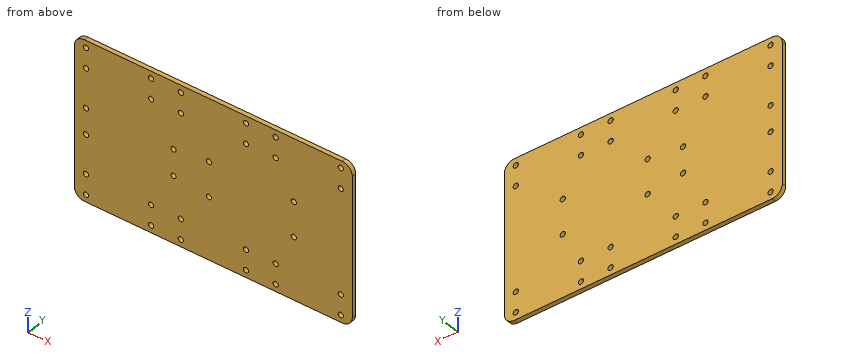
from build123d import *

# Parameters (mm, degrees)
SKETCH1_W            = 190
SKETCH1_H            = 110
BOSS_EXTRUDE1_DEPTH  = 3
M3_CLEARANCE_HOLE1_D = 3.6
FILLET1_R            = 7


with BuildPart() as part:
    # Sketch1 → Boss-Extrude1 (new body)
    with BuildSketch(Plane(origin=(0, 0, 0), x_dir=(1, 0, 0), z_dir=(0, 1, 0))):
        with Locations((95, 55)):
            Rectangle(SKETCH1_W, SKETCH1_H)
    extrude(amount=BOSS_EXTRUDE1_DEPTH)

    # M3 Clearance Hole1 (through all)
    with Locations(Plane(origin=(0, 3, 0), x_dir=(1, 0, 0), z_dir=(0, 1, 0))):
        with Locations((8, 105), (52.5, 105), (52.5, 91), (8, 91), (52.5, 19), (52.5, 5), (8, 19), (8, 5), (72.811, 105), (117.311, 105), (117.311, 91), (72.811, 91), (137.622, 105), (182.122, 105), (182.122, 91), (137.622, 91), (72.811, 19), (117.311, 19), (137.622, 19), (182.122, 19), (182.122, 5), (137.622, 5), (117.311, 5), (72.811, 5), (8, 64), (8, 46), (67.78, 64), (67.78, 46), (92, 67), (92, 43), (150, 43), (150, 67)):
            Hole(M3_CLEARANCE_HOLE1_D / 2)

    # Fillet1
    fillet1_edges = [part.edges().sort_by_distance(p)[0] for p in [
        (0, 1.5, -110),
        (190, 1.5, -110),
        (190, 1.5, 0),
        (0, 1.5, 0),
    ]]
    fillet(fillet1_edges, radius=FILLET1_R)


solid = part.part
For this review, take the finished solid that the model builds, in its own axes (mm). Round coordinates to 2 decimals unless told otherwise and drop trailing zeros. Order: outer loops, then holes, each group sorted by start corner. A loop starts at its lowest first (then second) coordinate and runs counter-clockwise, first axis right, second up. Notation, with made-up numbers: (-31, 36.5) -> (-15, 36.5) arc R21 cw to (-15, 66.5) -> close; hole circle Ø7 at (-4, 87). An arc over 180 degrees is marked (long way). Put each result on its own line as item: value.
Q1. For probe 1 along Z at (x, y) = (73, 0.8); probe 2 along X at (y, z) = (1.6, -67); probe 3 along X at (y, z) = (2.3, -64), list the stretches that pass through material, from the lowest coordinate up. Write a range as [from, to].
Check result:
probe 1: [-110, -106.79], [-103.21, -92.79], [-89.21, -20.79], [-17.21, -6.79], [-3.21, 0]
probe 2: [0, 90.2], [93.8, 148.2], [151.8, 190]
probe 3: [0, 6.2], [9.8, 65.98], [69.58, 190]
Q2. Add section D-D on z = -105. Write out the cut boundary in (x, y).
Check result:
outline: (0.29, 0) -> (6.2, 0) -> (6.2, 3) -> (0.29, 3) -> close; (9.8, 0) -> (50.7, 0) -> (50.7, 3) -> (9.8, 3) -> close; (54.3, 0) -> (71.01, 0) -> (71.01, 3) -> (54.3, 3) -> close; (74.61, 0) -> (115.51, 0) -> (115.51, 3) -> (74.61, 3) -> close; (119.11, 0) -> (135.82, 0) -> (135.82, 3) -> (119.11, 3) -> close; (139.42, 0) -> (180.32, 0) -> (180.32, 3) -> (139.42, 3) -> close; (183.92, 0) -> (189.71, 0) -> (189.71, 3) -> (183.92, 3) -> close
Q3. Add section A-A on z = -19. Write out the cut boundary in (x, y).
Check result:
outline: (0, 0) -> (6.2, 0) -> (6.2, 3) -> (0, 3) -> close; (9.8, 0) -> (50.7, 0) -> (50.7, 3) -> (9.8, 3) -> close; (54.3, 0) -> (71.01, 0) -> (71.01, 3) -> (54.3, 3) -> close; (74.61, 0) -> (115.51, 0) -> (115.51, 3) -> (74.61, 3) -> close; (119.11, 0) -> (135.82, 0) -> (135.82, 3) -> (119.11, 3) -> close; (139.42, 0) -> (180.32, 0) -> (180.32, 3) -> (139.42, 3) -> close; (183.92, 0) -> (190, 0) -> (190, 3) -> (183.92, 3) -> close
Q4. Add section C-C on y = 1.2. State how many separate pieces and enclosed holes the cut face has, plus the area to 3 significant figures.
Check result:
separate pieces: 1
enclosed holes: 32
area: 20,500 mm2
Q5. Add section B-B on x = 52.5. Write out the cut boundary in (y, z), plus the area to 3 significant figures.
Check result:
outline: (0, -110) -> (3, -110) -> (3, -106.8) -> (0, -106.8) -> close; (0, -103.2) -> (3, -103.2) -> (3, -92.8) -> (0, -92.8) -> close; (0, -89.2) -> (3, -89.2) -> (3, -20.8) -> (0, -20.8) -> close; (0, -17.2) -> (3, -17.2) -> (3, -6.8) -> (0, -6.8) -> close; (0, -3.2) -> (3, -3.2) -> (3, 0) -> (0, 0) -> close
area: 287 mm2
